```python
from build123d import *
from OCP.BRepFilletAPI import BRepFilletAPI_MakeChamfer

# Parameters (mm, degrees)
SKETCH3_W             = 46
SKETCH3_H             = 32
BOSS_EXTRUDE1_DEPTH   = 11.25
SKETCH5_R             = 6
SKETCH5_R_2           = 3.825
BOSS_EXTRUDE2_DEPTH   = 1.5
MOVE_FACE1_BY         = 0.5
MOVE_FACE1_2_BY       = 0.5
MOVE_FACE1_3_BY       = 0.5
MOVE_FACE1_4_BY       = 0.5
SKETCH6_R             = 3
BOSS_EXTRUDE3_DEPTH   = 14
SKETCH7_W             = 3.6
SKETCH7_H             = 0.6
CUT_EXTRUDE1_DEPTH    = 12
M3_TAPPED_HOLE1_D     = 2.5
M3_TAPPED_HOLE1_DEPTH = 8.5
M3_TAPPED_HOLE1_TIP   = 0.751075774
M3_TAPPED_HOLE2_D     = 2.5
M3_TAPPED_HOLE2_DEPTH = 8.5
M3_TAPPED_HOLE2_TIP   = 0.751075774
CHAMFER1_SIZE         = 2
CHAMFER1_SIZE2        = 7.464101615
SKETCH13_R            = 12.2
BOSS_EXTRUDE4_DEPTH   = 30.5
SKETCH14_R            = 3.175
BOSS_EXTRUDE6_DEPTH   = 1.5


with BuildPart() as part:
    # Sketch3 → Boss-Extrude1 (new, symmetric)
    with BuildSketch(Plane.XY):
        with Locations((8, 0)):
            Rectangle(SKETCH3_W, SKETCH3_H)
    extrude(amount=BOSS_EXTRUDE1_DEPTH, both=True)

    # Sketch5 → Boss-Extrude2 (add)
    with BuildSketch(Plane.XY.offset(11.25)):
        Circle(SKETCH5_R)
        with Locations((-9, 9)):
            Circle(SKETCH5_R_2)
        with Locations((-9, -9)):
            Circle(SKETCH5_R_2)
        with Locations((24, 9)):
            Circle(SKETCH5_R_2)
        with Locations((24, -9)):
            Circle(SKETCH5_R_2)
    extrude(amount=BOSS_EXTRUDE2_DEPTH)

    # Move Face1: a face moved outward by 0.5
    extrude(part.faces().sort_by_distance((24, -9, 12.75))[0], amount=MOVE_FACE1_BY, dir=(0, 0, 1))

    # Move Face1 2: a face moved outward by 0.5
    extrude(part.faces().sort_by_distance((24, 9, 12.75))[0], amount=MOVE_FACE1_2_BY, dir=(0, 0, 1))

    # Move Face1 3: a face moved outward by 0.5
    extrude(part.faces().sort_by_distance((-9, -9, 12.75))[0], amount=MOVE_FACE1_3_BY, dir=(0, 0, 1))

    # Move Face1 4: a face moved outward by 0.5
    extrude(part.faces().sort_by_distance((-9, 9, 12.75))[0], amount=MOVE_FACE1_4_BY, dir=(0, 0, 1))

    # Sketch6 → Boss-Extrude3 (add)
    with BuildSketch(Plane.XY.offset(12.75)):
        Circle(SKETCH6_R)
    extrude(amount=BOSS_EXTRUDE3_DEPTH)

    # Sketch7 → Cut-Extrude1 (cut)
    with BuildSketch(Plane.XY.offset(26.75)):
        with Locations((0, 2.7)):
            Rectangle(SKETCH7_W, SKETCH7_H)
    extrude(amount=-CUT_EXTRUDE1_DEPTH, mode=Mode.SUBTRACT)

    # M3 Tapped Hole1
    with Locations(Plane.XY.offset(13.25)):
        with Locations((-9, 9), (-9, -9), (24, 9), (24, -9)):
            Hole(M3_TAPPED_HOLE1_D / 2, depth=M3_TAPPED_HOLE1_DEPTH)
            with Locations((0, 0, -(M3_TAPPED_HOLE1_DEPTH + M3_TAPPED_HOLE1_TIP / 2))):  # 118° drill point
                Cone(0, M3_TAPPED_HOLE1_D / 2, M3_TAPPED_HOLE1_TIP, mode=Mode.SUBTRACT)

    # M3 Tapped Hole2
    with Locations(Plane.XY.offset(26.75)):
        with Locations((0, 0)):
            Hole(M3_TAPPED_HOLE2_D / 2, depth=M3_TAPPED_HOLE2_DEPTH)
            with Locations((0, 0, -(M3_TAPPED_HOLE2_DEPTH + M3_TAPPED_HOLE2_TIP / 2))):  # 118° drill point
                Cone(0, M3_TAPPED_HOLE2_D / 2, M3_TAPPED_HOLE2_TIP, mode=Mode.SUBTRACT)

    # Chamfer1: one chamfer whose edges measure the first distance from different faces: ONE call of the kernel's chamfer builder (chamfer() names one face for all edges)
    chamfer1_edges_1 = [part.edges().sort_by_distance(p)[0] for p in [
        (8, 16, -11.25),
    ]]
    chamfer1_side_1 = [part.faces().sort_by_distance(p)[0] for p in [
        (8, 16, 0),
    ]]
    chamfer1_edges_2 = [part.edges().sort_by_distance(p)[0] for p in [
        (8, -16, -11.25),
    ]]
    chamfer1_side_2 = [part.faces().sort_by_distance(p)[0] for p in [
        (8, -16, 0),
    ]]
    chamfer1 = BRepFilletAPI_MakeChamfer(part.part.solid().wrapped)
    for e in chamfer1_edges_1:
        chamfer1.Add(CHAMFER1_SIZE, CHAMFER1_SIZE2, e.wrapped, chamfer1_side_1[0].wrapped)  # the first distance lies on this face
    for e in chamfer1_edges_2:
        chamfer1.Add(CHAMFER1_SIZE, CHAMFER1_SIZE2, e.wrapped, chamfer1_side_2[0].wrapped)  # the first distance lies on this face
    add(Compound.cast(chamfer1.Shape()), mode=Mode.REPLACE)

    # Sketch13 → Boss-Extrude4 (add)
    with BuildSketch(Plane(origin=(31, 0, 0), x_dir=(0, 0, -1), z_dir=(1, 0, 0))):
        with Locations(Location((2, 3, 0), (0, 0, 319.305481692))):
            Circle(SKETCH13_R)
    extrude(amount=BOSS_EXTRUDE4_DEPTH)

    # Sketch14 → Boss-Extrude6 (add)
    with BuildSketch(Plane(origin=(61.5, 0, 0), x_dir=(0, 0, -1), z_dir=(1, 0, 0))):
        with Locations(Location((2, 3, 0), (0, 0, 90))):
            Circle(SKETCH14_R)
    extrude(amount=BOSS_EXTRUDE6_DEPTH)


solid = part.part
```
CAD build for the part. Positions are in the model's coordinates, mm. A direction names the side the tool comes from. Coordinates: 2 decimals unless noted, no trailing zeros. Order: outer loops, then holes, each group sorted by start corner. A loop starts at its lowest first (then second) coordinate and runs counter-clockwise, first axis right, second up. Notation, with made-up numbers: M -21,53 L 34,53 A19 cw 34,69 Z; hole C -1.75,46 d3. An arc over 180 degrees is marked long. Answer as CSV lines item,"result".
1) Flat gauge pins, fed straight in: P1, Ø2.5, axis at x = 24, y = 10.5, coming from the +Z side; P2, Ø4, axis at x = 0, z = 21, coming from the +Y side; P3, Ø10, axis at y = -6, z = 19.5, coming from the -X side. Where does each tip first touch, or does it go through?
Verdict:
P1,"z = 13.25"
P2,"y = 2.4"
P3,"x = -2.83"
2) Cut at D-D (y = -7). List the corners of the cut face in (x, z), then the cut area to 3 significant figures.
Verdict:
outline,"M -15,-11.25 L 31,-11.25 L 31,-8.99 L 61.5,-8.99 L 61.5,4.99 L 31,4.99 L 31,11.25 L 27.26,11.25 L 27.26,13.25 L 20.74,13.25 L 20.74,11.25 L -5.74,11.25 L -5.74,13.25 L -12.26,13.25 L -12.26,11.25 L -15,11.25 Z"
area,"1,490 mm2"
3) Cut at C-C (z = -2). List the corners of the cut face in (x, y) (3 decimals), then the cut area to 3 significant figures.
Verdict:
outline,"M -15,-16 L 31,-16 L 31,-9.2 L 61.5,-9.2 L 61.5,-0.175 L 63,-0.175 L 63,6.175 L 61.5,6.175 L 61.5,15.2 L 31,15.2 L 31,16 L -15,16 Z"
area,"2,230 mm2"
4) 3-axis set-ups, long thin cutter, end or side, ignore diameter. For faces 1 (the cylindrical face through (62.24, 0.48, -3.93)), 2 (the cylindrical face through (20.18, 9.17, 12.24)), 3 (the flat face through (8, -16, 1)): which of +Z, -Z, +X, -X, +Y, -Y reach the whole face in a straight line?
Verdict:
face 1,"+X"
face 2,"+Z"
face 3,"+Z, -Z, +X, -X, -Y"
5) Cut at A-A (z = 7.5). List the corners of the cut face in (x, y), then the cut area to 3 significant figures.
Verdict:
outline,"M -15,-16 L 31,-16 L 31,-4.65 L 61.5,-4.65 L 61.5,10.65 L 31,10.65 L 31,16 L -15,16 Z; hole C -9,-9 d2.5; hole C -9,9 d2.5; hole C 24,-9 d2.5; hole C 24,9 d2.5"
area,"1,920 mm2"
6) Mould opens along X. For faces 4 (the flat face through (31, -7.2, 5.1)), 5 (the conical face through (-0.05, -0.21, 17.63)), 6 (the flat face through (7.678, 12.216, -10.264)) say: released by +X, released by -X, zero draft, split by the parting line, or undercut.
Verdict:
face 4,"released by +X"
face 5,"undercut"
face 6,"zero draft"
7) Drill centre lines: L1, parallel to Y at x = 24, z = 9; L2, parallel to X at y = 9, z = 8; L3, parallel to X at y = 9, z = 11. Where is each one in solid material? Low to high. Write a range as from..to.
Verdict:
L1,"-16..-10.25, -7.75..7.75, 10.25..16"
L2,"-15..-10.25, -7.75..22.75, 25.25..61.5"
L3,"-15..-10.25, -7.75..22.75, 25.25..31"
8) Cut at B-B (x = 26). List the corners of the cut face in (y, z).
Verdict:
outline,"M -16,-9.25 L -8.54,-11.25 L 8.54,-11.25 L 16,-9.25 L 16,11.25 L 12.26,11.25 L 12.26,13.25 L 5.74,13.25 L 5.74,11.25 L -5.74,11.25 L -5.74,13.25 L -12.26,13.25 L -12.26,11.25 L -16,11.25 Z"
